```python
from build123d import *

# Parameters (mm, degrees)
CROQUIS1_R              = 3
SALIENTE_EXTRUIR1_DEPTH = 3
CROQUIS2_W              = 33
CROQUIS2_H              = 30
CORTAR_EXTRUIR2_DEPTH   = 3


with BuildPart() as part:
    # Croquis1 → Saliente-Extruir1 (new body)
    with BuildSketch(Plane(origin=(0, 0, 0), x_dir=(1, 0, 0), z_dir=(0, 1, 0))):
        Polygon((182, 120), (205, 120), (205, -120), (-205, -120), (-205, 120), (-182, 120), (-182, 140), (-25, 140), (-25, 122), (25, 122), (25, 140), (182, 140), align=None)
        with Locations(Location((-195, 110, 0), (0, 0, 270))):
            Circle(CROQUIS1_R, mode=Mode.SUBTRACT)
        with Locations(Location((-195, 0, 0), (0, 0, 270))):
            Circle(CROQUIS1_R, mode=Mode.SUBTRACT)
        with Locations(Location((-195, -110, 0), (0, 0, 90))):
            Circle(CROQUIS1_R, mode=Mode.SUBTRACT)
        with Locations(Location((195, -110, 0), (0, 0, 270))):
            Circle(CROQUIS1_R, mode=Mode.SUBTRACT)
        with Locations(Location((195, 0, 0), (0, 0, 90))):
            Circle(CROQUIS1_R, mode=Mode.SUBTRACT)
        with Locations(Location((195, 110, 0), (0, 0, 90))):
            Circle(CROQUIS1_R, mode=Mode.SUBTRACT)
        with Locations(Location((0, -110, 0), (0, 0, 270))):
            Circle(CROQUIS1_R, mode=Mode.SUBTRACT)
        with Locations(Location((144.549746064, 130, 0), (0, 0, 270))):
            Circle(CROQUIS1_R, mode=Mode.SUBTRACT)
        with Locations(Location((-144.549746064, 130, 0), (0, 0, 90))):
            Circle(CROQUIS1_R, mode=Mode.SUBTRACT)
    extrude(amount=SALIENTE_EXTRUIR1_DEPTH)

    # Croquis2 → Cortar-Extruir2 (cut)
    with BuildSketch(Plane(origin=(0, 3, 0), x_dir=(1, 0, 0), z_dir=(0, 1, 0))):
        with Locations((123.996419689, -84)):
            Rectangle(CROQUIS2_W, CROQUIS2_H)
    extrude(amount=-CORTAR_EXTRUIR2_DEPTH, mode=Mode.SUBTRACT)


solid = part.part
```
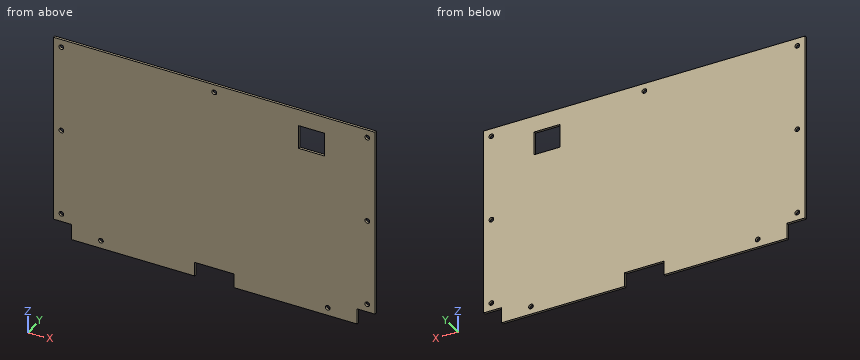
Check sheet for the modelled part. Datum: model origin and axes. Units: mm. Round coordinates to 2 decimals unless told otherwise and drop trailing zeros. Order: outer loops, then holes, each group sorted by start corner. A loop starts at its lowest first (then second) coordinate and runs counter-clockwise, first axis right, second up. Notation, with made-up numbers: (-6, 82) - (16, 82) arc R15 ccw to (16, 98) - close; hole circle Ø1 at (67, -38.75). An arc over 180 degrees is marked (long way). Answer as CSV lines item,"result". Start each with the question number.
1) Scan lines: probe 1 along X at (y, z) = (2, 110); probe 2 along X at (y, z) = (1.3, -130); probe 3 along X at (y, z) = (0.5, -0.5). Record each from-to range of solid material in increasing order.
2) Section check B-B (y = 2.2). Give the number of separate pieces and of enclosed holes in the cut face, then the cut area to 3 significant figures.
3) Depth check by flat-ended pin: pin 1 (0.9 mm diameter, centred on y = 1.5, z = -128, fed in from +X); pin 2 (1.5 mm diameter, centred on x = 2.5, y = 1.5, fed in from -Z). Enter the tip coordinate at first touch or a pass-through.
4) Section check A-A (z = 74). Record the cut outline in (x, y).
Determined:
1,probe 1,"-205 to -198, -192 to -3, 3 to 192, 198 to 205"
1,probe 2,"-182 to -147.55, -141.55 to -25, 25 to 141.55, 147.55 to 182"
1,probe 3,"-205 to -197.96, -192.04 to 192.04, 197.96 to 205"
2,separate pieces,"1"
2,enclosed holes,"10"
2,area,"104,000 mm^2"
3,pin 1,"x = 182"
3,pin 2,"z = -122"
4,outline,"(-205, 0) - (107.5, 0) - (107.5, 3) - (-205, 3) - close; (140.5, 0) - (205, 0) - (205, 3) - (140.5, 3) - close"
